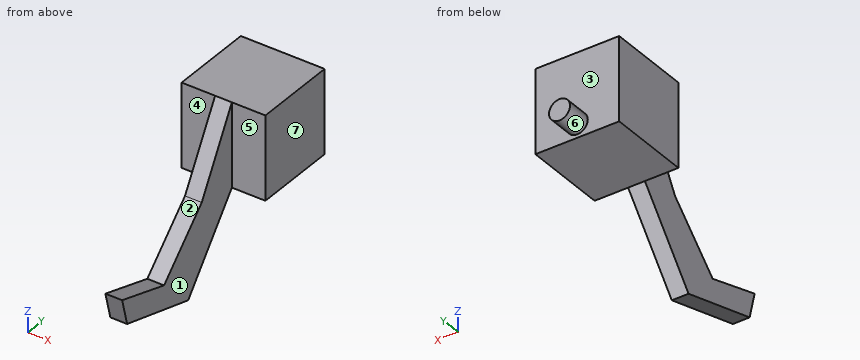
```python
from build123d import *

# Parameters (mm, degrees)
F0_W     = 25.4
F0_H     = 25.4
F1_DEPTH = 25.4
F4_DEPTH = 5.08
F5_R     = 3.175
F6_DEPTH = 7.62


with BuildPart() as f1:
    # F0 (on Top) → F1 (new body)
    with BuildSketch(Plane.XY):
        with Locations((0, 12.7)):
            Rectangle(F0_W, F0_H)
    extrude(amount=F1_DEPTH)

    # F3 (on offset) → F4 (join)
    with BuildSketch(Plane.YZ.offset(2.54)):
        Polygon((-18.736662, -23.311928), (0, 0), (0, 25.4), (-12.919935, 2.629027), (-29.085293, -13.219362), (-47.073215, -7.830909), (-44.933684, -16.072072), align=None)
    extrude(amount=-F4_DEPTH)

    # F5 (on face) → F6 (join)
    with BuildSketch(Plane(origin=(0, 25.4, 0), x_dir=(-1, 0, 0), z_dir=(0, 1, 0))):
        with Locations((0, 4.182435)):
            Circle(F5_R)
    extrude(amount=F6_DEPTH)


solid = f1.part
```
Here's how the part is built. I have some questions about the finished solid (model axes, mm). Face numbers are marked on the shaded views. A direction names the side the tool comes from. Round coordinates to 2 decimals unless told otherwise and drop trailing zeros. Order: outer loops, then holes, each group sorted by start corner. A loop starts at its lowest first (then second) coordinate and runs counter-clockwise, first axis right, second up. Notation, with made-up numbers: M 68.5,1 L 99.5,1 A24 ccw 99.5,36 Z; hole C 9,41 d5. An arc over 180 degrees is marked long. Answer as CSV lines item,"result".
Item 1: For pin 1 (1.5 mm diameter, centred on x = 1.5, y = -20, fed in from +Z); pin 2 (2 mm diameter, centred on x = 3, y = -28.5, fed in from -Z); pin 3 (23.5 mm diameter, centred on y = -24.5, z = -5, fed in from +X), each with a flat end and sliding along its axis, tell me the tip position at first contact or that it passes through.
From the geometry:
pin 1,"z = -3.58"
pin 2,"z = -20.86"
pin 3,"x = 2.54"
Item 2: Imagine slicing it at C-C on y = 23. List the corners of the cut face in (x, z) for me, and give its area (3 significant figures).
From the geometry:
outline,"M -12.7,0 L 12.7,0 L 12.7,25.4 L -12.7,25.4 Z"
area,"645 mm2"
Item 3: Which directions (+Z, -Z, +X, -X, +Y, -Y) give clear straight access to the entire face, cutting with the end or side of a thin tool? Please do the marked faces 4, 5, 6 and 7.
From the geometry:
face 4,"+Z, -Z, -X, -Y"
face 5,"+Z, -Z, +X, -Y"
face 6,"+Y"
face 7,"+Z, -Z, +X, +Y, -Y"
Item 4: We'd pull the mould along Y, two halves only. Please class the marked faces 1, 2 and 3: +Y half, -Y half, draft (parallel to the pull), parting line (faces both ways), or undercut.
From the geometry:
face 1,"draft"
face 2,"undercut"
face 3,"+Y half"
Item 5: Imagine slicing it at A-A on x = 0. List the corners of the cut face in (y, z) for me, and give its area (3 significant figures).
From the geometry:
outline,"M -47.07,-7.83 L -44.93,-16.07 L -18.74,-23.31 L 0,0 L 25.4,0 L 25.4,1.01 L 33.02,1.01 L 33.02,7.36 L 25.4,7.36 L 25.4,25.4 L 0,25.4 L -12.92,2.63 L -29.09,-13.22 Z"
area,"1,360 mm2"
Item 6: Please list where these lines run through material, in increasing order: L1, parallel to Z at x = 5.75, y = 10.5; L2, parallel to X at y = -8.5, z = 6.5. Write a range as [from, to].
From the geometry:
L1,"[0, 25.4]"
L2,"[-2.54, 2.54]"
Item 7: Imagine slicing it at B-B on z = 17. List the corners of the cut face in (x, y) for me, and give its area (3 significant figures).
From the geometry:
outline,"M -12.7,0 L -2.54,0 L -2.54,-4.77 L 2.54,-4.77 L 2.54,0 L 12.7,0 L 12.7,25.4 L -12.7,25.4 Z"
area,"669 mm2"
Item 8: Imagine slicing it at D-D on x = -7.75. List the corners of the cut face in (y, z) for me, and give its area (3 significant figures).
From the geometry:
outline,"M 0,0 L 25.4,0 L 25.4,25.4 L 0,25.4 Z"
area,"645 mm2"
